```python
from build123d import *

# Parameters (mm, degrees)
SKETCH2_R           = 44.45
SKETCH2_R_2         = 38.1
BOSS_EXTRUDE1_DEPTH = 152.4
CUT_EXTRUDE1_DEPTH  = 152.4
SKETCH5_W           = 20.435442018
SKETCH5_H           = 152.4
BOSS_EXTRUDE2_DEPTH = 6.35
SKETCH6_W           = 8.676407007
SKETCH6_H           = 152.4
BOSS_EXTRUDE3_DEPTH = 63.5
SKETCH7_W           = 20.435442018
SKETCH7_H           = 152.4
BOSS_EXTRUDE4_DEPTH = 101.6


with BuildPart() as part:
    # Sketch2 → Boss-Extrude1 (new body)
    with BuildSketch(Plane.XY):
        Circle(SKETCH2_R)
        Circle(SKETCH2_R_2, mode=Mode.SUBTRACT)
    extrude(amount=BOSS_EXTRUDE1_DEPTH)

    # Sketch3 → Cut-Extrude1 (cut)
    with BuildSketch(Plane.XY.offset(152.4)):
        Polygon((-26.531587494, -35.663389702), (40.024531053, 19.334927308), (75.854578195, -15.638849725), (-9.866811461, -86.474293044), align=None)
    extrude(amount=-CUT_EXTRUDE1_DEPTH, mode=Mode.SUBTRACT)

    # Sketch5 → Boss-Extrude2 (add)
    with BuildSketch(Plane(origin=(6.746471779, -8.164231197, 0), x_dir=(-0.770864065, -0.63699968, 0), z_dir=(0.63699968, -0.770864065, 0))):
        with Locations((-46.816087742, -76.2)):
            Rectangle(SKETCH5_W, SKETCH5_H)
    extrude(amount=BOSS_EXTRUDE2_DEPTH)

    # Sketch6 → Boss-Extrude3 (add)
    with BuildSketch(Plane(origin=(6.746471779, -8.164231197, 0), x_dir=(0.770864065, 0.63699968, 0), z_dir=(-0.63699968, 0.770864065, 0))):
        with Locations((52.695605247, -76.2)):
            Rectangle(SKETCH6_W, SKETCH6_H)
    extrude(amount=BOSS_EXTRUDE3_DEPTH)

    # Sketch7 → Boss-Extrude4 (add)
    with BuildSketch(Plane(origin=(10.791419749, -13.059218012, 0), x_dir=(0.770864065, 0.63699968, 0), z_dir=(0.63699968, -0.770864065, 0))):
        with Locations((46.816087742, 76.2)):
            Rectangle(SKETCH7_W, SKETCH7_H)
    extrude(amount=BOSS_EXTRUDE4_DEPTH)


solid = part.part
```
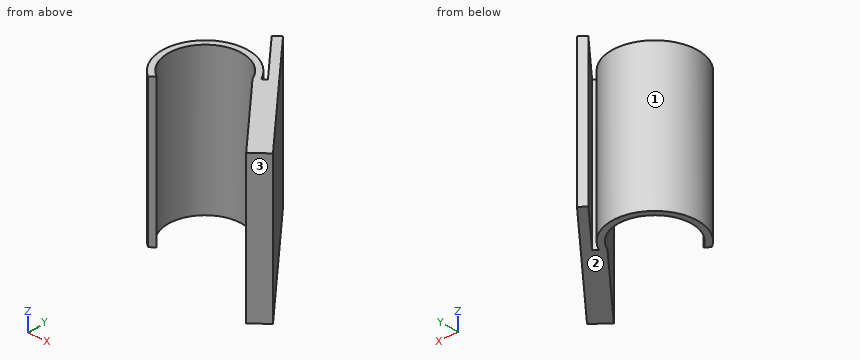
Geometry check sheet. Reference: the model listing, model coordinates, mm. Face numbers are marked on the shaded views. Coordinates: 2 decimals unless noted, no trailing zeros. Order: outer loops, then holes, each group sorted by start corner. A loop starts at its lowest first (then second) coordinate and runs counter-clockwise, first axis right, second up.
Q1. Sectioned sample at C-C on y = 31. Record the cut outline in (x, z).
Reply:
outline: (-31.86, 0) - (-22.15, 0) - (-22.15, 152.4) - (-31.86, 152.4) - close; (22.15, 0) - (31.86, 0) - (31.86, 152.4) - (22.15, 152.4) - close; (37.11, 0) - (48.37, 0) - (48.37, 152.4) - (37.11, 152.4) - close
Q2. Depth check by flat-ended pin: pin 1 Ø12 at (x, z) = (59, 122) entering from -Y; pin 2 Ø3 at (y, z) = (-36, 34) entering from +X; pin 3 Ø12 at (x, z) = (-18, 69) entering from -Y. Enter the tip coordinate at first touch or a pass-through.
Reply:
pin 1: stops at y = -21.21
pin 2: stops at x = 104.97
pin 3: stops at y = -33.57
Q3. Sectioned sample at B-B on x = 32.5. Record the cut outline in (y, z).
Reply:
outline: (19.88, 0) - (30.32, 0) - (30.32, 152.4) - (19.88, 152.4) - close; (36.58, 0) - (50.21, 0) - (50.21, 152.4) - (36.58, 152.4) - close
Q4. Sectioned sample at D-D on y = 0. Record the cut outline in (x, z), and give its area (3 significant figures).
Reply:
outline: (-44.45, 0) - (-38.1, 0) - (-38.1, 152.4) - (-44.45, 152.4) - close; (47.48, 0) - (73.99, 0) - (73.99, 152.4) - (47.48, 152.4) - close
area: 5,010 mm2
Q5. Sectioned sample at A-A on z = 26. Record the cut outline in (x, y), and give its area (3 significant figures).
Reply:
outline: (-26.53, -35.66) - (-21.47, -31.48) arc R38.1 cw (long way) to (34.96, 15.15) - (103.72, -68.07) - (119.48, -55.05) - (10.26, 77.12) - (3.57, 71.59) - (44.02, 22.64) - (40.02, 19.33) arc R44.45 ccw (long way) to start
area: 3,720 mm2
Q6. Thickness scan on probe 1 along X at (y, z) = (31.5, 28); probe 2 along Y at (x, z) = (0, 96.5); probe 3 along Y at (x, z) = (-32, 74.5). Record the ranges inside material, lowest first.
Reply:
probe 1: x = -31.36 to -21.43, 21.43 to 31.36, 36.7 to 47.96
probe 2: y = 38.1 to 44.45
probe 3: y = -30.85 to -20.68, 20.68 to 30.85
Q7. Draft check along Y on the marked faces 1, 2 and 3. Enter one of: released by +Y, released by -Y, zero draft, split by the parting line, or undercut.
Reply:
face 1: undercut
face 2: zero draft
face 3: released by -Y
